Build history of the part. All positions in model axes, mm. Face numbers are marked on the shaded views. A direction names the side the tool comes from. Give positions to 0.01 mm unless a question says otherwise; leave off trailing zeros. Write each loop counter-clockwise with the first axis right and the second up, starting at its lowest first coordinate (ties: lowest second). Pieces come first, ordered by that corner, then holes. Notation, with made-up numbers: M 81,-5 L 88,-5 A18 cw 88,7 Z; hole C 86,62.25 d10. An arc over 180 degrees is marked long. One line per item, written item: value. Start each with the question number.
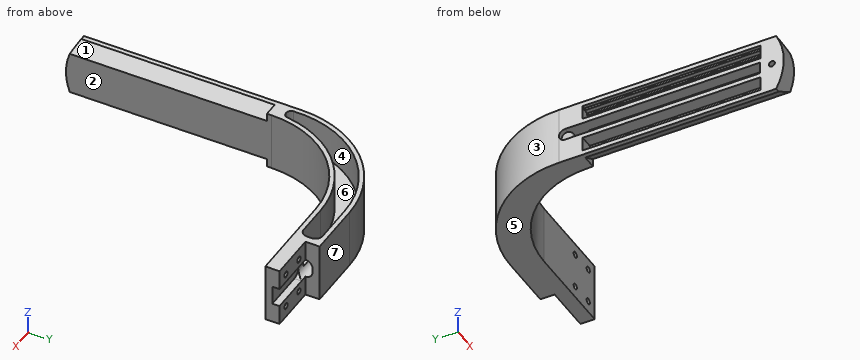
from build123d import *

# Parameters (mm, degrees)
EXTRUDE_1_DEPTH      = 25
SKETCH_2_W           = 20.000000000000014
SKETCH_2_H           = 6
CUT_EXTRUDE_1_DEPTH  = 168.23934943666816
CUT_EXTRUDE_2_DEPTH  = 85
CUT_EXTRUDE_4_DEPTH  = 5
CUT_EXTRUDE_3_REACH  = 169.239
FILLET_3_R           = 2
FILLET_4_R           = 3
CUT_EXTRUDE_6_DEPTH  = 75
M3X0_51_D            = 2.5
CUT_EXTRUDE_7_REACH  = 169.239
CUT_EXTRUDE_8_DEPTH  = 3
FILLET_8_R           = 3
CUT_EXTRUDE_9_DEPTH  = 28
CUT_EXTRUDE_10_DEPTH = 6
EXTRUDE_2_DEPTH      = 5
M3X0_52_D            = 2.5
M3X0_52_DEPTH        = 4
M3X0_52_TIP          = 0.7510757737844503


with BuildPart() as part:
    # Эскиз1 → Бобышка-Вытянуть1 (new body)
    with BuildSketch(Plane.XY):
        with BuildLine():
            Line((0, 0), (0, 95))
            ThreePointArc((0, 95), (13.18019484660537, 126.81980515339464), (45, 140))
            Line((45, 140), (88, 140))
            Line((88, 140), (88, 128))
            Line((88, 128), (49, 127.99999999999997))
            ThreePointArc((49, 127.99999999999997), (20.00862197135158, 115.99137802864843), (8.000000000000002, 87))
            Line((8.000000000000002, 87), (8, 0))
            Line((8, 0), (0, 0))
        make_face()
    extrude(amount=EXTRUDE_1_DEPTH)

    # Эскиз2 → Вырез-Вытянуть1 (cut, through all)
    with BuildSketch(Plane.XY.offset(25)):
        with Locations((78, 137)):
            Rectangle(SKETCH_2_W, SKETCH_2_H)
    extrude(amount=-CUT_EXTRUDE_1_DEPTH, mode=Mode.SUBTRACT)

    # Эскиз5 → Вырез-Вытянуть2 (cut)
    with BuildSketch(Plane.XZ):
        Polygon((8, 3.4641016151377366), (2, 0), (8, 0), (10.194072484648698, 0), (10.1940724846487, 4.730849954771208), align=None)
        Polygon((1.9999999999999971, 25), (7.999999999999993, 25), (10.194072484648695, 25), (10.194072484648698, 20.26915004522879), (7.999999999999998, 21.535898384862264), align=None)
    extrude(amount=-CUT_EXTRUDE_2_DEPTH, mode=Mode.SUBTRACT)

    # Эскиз6 → Вырез-Вытянуть4 (cut)
    with BuildSketch(Plane.ZY):
        with BuildLine():
            Line((10.000000000000004, -11.916065179701535), (10.000000000000004, 92.5))
            ThreePointArc((10.000000000000004, 92.5), (12.500000000000004, 95), (15.000000000000005, 92.5))
            Line((15.000000000000005, 92.5), (15.000000000000005, -11.916065179701535))
            ThreePointArc((15.000000000000005, -11.916065179701535), (12.500000000000004, -14.416065179701535), (10.000000000000004, -11.916065179701535))
        make_face()
    extrude(amount=-CUT_EXTRUDE_4_DEPTH, mode=Mode.SUBTRACT)

    # Вырез-Вытянуть3: up to this face of the body (flat: up to its plane)
    cut_extrude_3_end = Plane(part.part.faces().sort_by_distance((2.5, 46.25, 10))[0])
    # Эскиз3 → Вырез-Вытянуть3 (cut, up to the picked face)
    with BuildSketch(Plane(origin=(0, 0, 25), x_dir=(-1, 0, 0), z_dir=(0, 0, -1)), mode=Mode.PRIVATE) as cut_extrude_3_sk1:
        with BuildLine():
            Line((-64.99999999999999, 138), (-64.99999999999999, 130))
            Line((-64.99999999999999, 130), (-49.00000000000001, 130))
            ThreePointArc((-49.00000000000001, 130), (-20.04313552885945, 118.78836265050464), (-6.186450742784722, 90.9999999999999))
            Line((-6.186450742784722, 90.9999999999999), (-2.186450742784722, 90.9999999999999))
            ThreePointArc((-2.186450742784722, 90.9999999999999), (-13.211637349495152, 123.9568644711403), (-44.999999999999545, 138))
            Line((-44.999999999999545, 138), (-64.99999999999999, 138))
        make_face()
    cut_extrude_3_tool1 = split(extrude(cut_extrude_3_sk1.sketch, amount=CUT_EXTRUDE_3_REACH, mode=Mode.PRIVATE), bisect_by=cut_extrude_3_end, keep=Keep.BOTH, mode=Mode.PRIVATE)
    add(cut_extrude_3_tool1.solids().sort_by(Axis((55, 137.213997, 25), (0, 0, -1)))[0], mode=Mode.SUBTRACT)

    # Скругление3
    fillet_3_edges = [part.edges().sort_by_distance(p)[0] for p in [
        (6.186450742784729, 90.9999999999999, 17.5),
        (2.186450742784718, 90.9999999999999, 20.000000000000004),
    ]]
    fillet(fillet_3_edges, radius=FILLET_3_R)

    # Скругление4
    fillet_4_edges = [part.edges().sort_by_distance(p)[0] for p in [
        (64.99999999999999, 138, 17.5),
        (64.99999999999999, 130, 17.5),
    ]]
    fillet(fillet_4_edges, radius=FILLET_4_R)

    # Эскиз8 → Вырез-Вытянуть6 (cut)
    with BuildSketch(Plane(origin=(0, 10, 0), x_dir=(1, 0, 0), z_dir=(0, 1, 0))):
        Polygon((0, -2), (1.5, -2), (1.5, -3), (3.4999999999999996, -3), (3.4999999999999996, -4.0000000000000036), (5.499999999999993, -4.0000000000000036), (5.499999999999994, -8.000000000000004), (0, -8.000000000000004), align=None)
        Polygon((3.500000000000003, -22.000000000000004), (3.500000000000003, -20.999999999999996), (5.499999999999995, -20.999999999999996), (5.499999999999996, -16.999999999999996), (6.94e-15, -16.999999999999996), (6.94e-15, -23), (1.5000000000000036, -23), (1.5000000000000036, -22.000000000000004), align=None)
    extrude(amount=CUT_EXTRUDE_6_DEPTH, mode=Mode.SUBTRACT)

    # Отверстие обработанное метчиком M3x0.51 (through all)
    with Locations(Plane(origin=(19.191951444358242, 134, 18.79968596761044), x_dir=(1, 0, 0), z_dir=(0, 1, 0))):
        with Locations((53.808048556, 13.799685968), (63.808048556, 13.799685968), (63.808048556, -1.200314032), (53.808048556, -1.200314032)):
            Hole(M3X0_51_D / 2)

    # Эскиз12 → Вырез-Вытянуть7 (cut, up to next)
    with BuildSketch(Plane.ZY, mode=Mode.PRIVATE) as cut_extrude_7_sk1:
        with BuildLine():
            Line((0, 3.301973769644008), (0, 0))
            Line((0, 0), (12.500000000000004, -3.47e-15))
            Line((12.500000000000004, -3.47e-15), (25, 0))
            Line((25, 0), (25, 3.301973769644008))
            ThreePointArc((25, 3.301973769644008), (12.500000000000005, 0.10000000000000142), (0, 3.301973769644008))
        make_face()
    cut_extrude_7_tool1 = extrude(cut_extrude_7_sk1.sketch, amount=-CUT_EXTRUDE_7_REACH, mode=Mode.PRIVATE) & part.part
    add(cut_extrude_7_tool1.solids().sort_by_distance((0, 1.650987, 0.252171))[0], mode=Mode.SUBTRACT)

    # Эскиз13 → Вырез-Вытянуть8 (cut)
    with BuildSketch(Plane(origin=(0, 134, 0), x_dir=(1, 0, 0), z_dir=(0, 1, 0))):
        Polygon((68.00000000000009, -8.5), (88.00000000000001, -8.499999999999996), (88.00000000000001, -16.5), (68.00000000000009, -16.499999999999996), align=None)
    extrude(amount=-CUT_EXTRUDE_8_DEPTH, mode=Mode.SUBTRACT)

    # Скругление8
    fillet_8_edges = [part.edges().sort_by_distance(p)[0] for p in [
        (68.00000000000009, 132.5, 16.499999999999996),
        (68.00000000000009, 132.5, 8.5),
    ]]
    fillet(fillet_8_edges, radius=FILLET_8_R)

    # Эскиз14 → Вырез-Вытянуть9 (cut)
    with BuildSketch(Plane(origin=(88, 0, 0), x_dir=(0, 0, -1), z_dir=(1, -1.16e-15, 0))):
        with BuildLine():
            Line((-13.499999999999998, 137), (-11.5, 137))
            ThreePointArc((-11.5, 137), (-8.5, 134), (-11.5, 131))
            Line((-11.5, 131), (-13.499999999999998, 131))
            ThreePointArc((-13.499999999999998, 131), (-16.5, 134), (-13.499999999999998, 137))
        make_face()
    extrude(amount=-CUT_EXTRUDE_9_DEPTH, mode=Mode.SUBTRACT)

    # Эскиз15 → Вырез-Вытянуть10 (cut)
    with BuildSketch(Plane.ZY):
        with BuildLine():
            Line((15.000000000000004, 92.5), (15.000000000000004, 85.49999999999999))
            ThreePointArc((15.000000000000004, 85.49999999999999), (12.500000000000005, 82.99999999999999), (10.000000000000007, 85.49999999999999))
            Line((10.000000000000007, 85.49999999999999), (10.000000000000005, 92.5))
            ThreePointArc((10.000000000000005, 92.5), (12.500000000000004, 95), (15.000000000000004, 92.5))
        make_face()
    extrude(amount=-CUT_EXTRUDE_10_DEPTH, mode=Mode.SUBTRACT)

    # Эскиз19 → Бобышка-Вытянуть2 (add)
    with BuildSketch(Plane.ZY):
        with BuildLine():
            Line((10.000000000000002, 10.100000000000001), (10.000000000000004, 0.22047141078493024))
            ThreePointArc((10.000000000000004, 0.22047141078493024), (12.500000000000005, 0.09999999999999787), (15.000000000000004, 0.22047141078493718))
            Line((15.000000000000004, 0.22047141078493718), (15.000000000000002, 10.100000000000001))
            Line((15.000000000000002, 10.100000000000001), (10.000000000000002, 10.100000000000001))
        make_face()
    extrude(amount=-EXTRUDE_2_DEPTH)

    # Отверстие обработанное метчиком M3x0.52
    with Locations(Plane.ZY):
        with Locations((12.5, 5.1)):
            Hole(M3X0_52_D / 2, depth=M3X0_52_DEPTH)
            with Locations((0, 0, -(M3X0_52_DEPTH + M3X0_52_TIP / 2))):  # 118° drill point
                Cone(0, M3X0_52_D / 2, M3X0_52_TIP, mode=Mode.SUBTRACT)


solid = part.part
1) Drop flat-ended pins along their axis: P1, Ø4.5, axis at x = 54, z = 15.5, coming from the -Y side; P2, Ø1.6, axis at y = 134.5, z = 23, coming from the -X side; P3, Ø5, axis at y = 83.5, z = 9, coming from the +X side; P4, Ø5, axis at x = 2.5, y = 33, coming from the -Z side. Give the stop position or say it passes through.
2) Mould opens along Y. For the marked faces 4, 5, 6 and 7 say: released by +Y, released by -Y, zero draft, split by the parting line, or undercut.
3) Band-saw the part on B-B (x = 27). List the corners of the cut face in (y, z), then the cut area to 3 significant figures.
4) Band-saw the part on C-C (y = 97.5). List the corners of the cut face in (x, z), then the cut area to 3 significant figures.
5) Tool access for the marked faces 1, 2 and 3: list every direction of +Z, -Z, +X, -X, +Y, -Y with a clear straight run to the whole face (end or side of a thin tool).
6) Band-saw the part on A-A (y = 63). List the corners of the cut face in (x, z).
7) Probe line 1 along Z through (x, y) = (83, 129.9); line 2 along Z through (x, y) = (83, 131.15); line 3 along X through (y, z) = (130.2, 5). List the from-to ranges inside material, lowest first. Write a range as from..to.
Model answer:
1. P1: stops at y = 128
1. P2: stops at x = 22.04
1. P3: stops at x = 8
1. P4: stops at z = 0
2. face 4: undercut
2. face 5: zero draft
2. face 6: undercut
2. face 7: released by +Y
3. outline: M 121.6,0 L 136.24,0 L 136.24,25 L 134.05,25 L 134.05,10 L 123.95,10 L 123.95,25 L 121.6,25 Z
3. area: 215 mm²
4. outline: M 0.07,0 L 9.37,0 L 9.37,25 L 7.3,25 L 7.3,10 L 2.07,10 L 2.07,25 L 0.07,25 Z
4. area: 154 mm²
5. face 1: +Z, +X, -Y
5. face 2: +Z, -Z, +X, -Y
5. face 3: +Z, -Z, -X, +Y
6. outline: M 0,0 L 2,0 L 8,3.46 L 8,21.54 L 2,25 L 0,25 L 0,23 L 1.5,23 L 1.5,22 L 3.5,22 L 3.5,21 L 5.5,21 L 5.5,17 L 0,17 L 0,15 L 5,15 L 5,10 L 0,10 L 0,8 L 5.5,8 L 5.5,4 L 3.5,4 L 3.5,3 L 1.5,3 L 1.5,2 L 0,2 Z
7. line 1: z = 0..3.75, 6.25..18.75, 21.25..25
7. line 2: z = 0..3.75, 6.25..8.5, 16.5..18.75, 21.25..25
7. line 3: x = 16.97..71.75, 74.25..81.75, 84.25..88
